Autodesk Fusion 360 part; units mm, degrees
sketch "Sketch3" plane through (0, 0, 18) normal (0, 0, 1) x (1, 0, 0)
  line L0 (-33.9, 6.35) -> (-19.5, 6.35) construction
  line L1 (-19.5, 6.35) -> (-19.5, -6.35) construction
  line L2 (-19.5, -6.35) -> (-33.9, -6.35) construction
  line L3 (-33.9, -6.35) -> (-33.9, 6.35) construction
  line L4 (19.5, 6.35) -> (33.9, 6.35) construction
  line L5 (33.9, 6.35) -> (33.9, -6.35) construction
  line L6 (33.9, -6.35) -> (19.5, -6.35) construction
  line L7 (19.5, -6.35) -> (19.5, 6.35) construction
  line L8 (-35.9, 8.35) -> (35.9, 8.35)
  line L9 (35.9, 8.35) -> (35.9, -8.35)
  line L10 (35.9, -8.35) -> (-35.9, -8.35)
  line L11 (-35.9, -8.35) -> (-35.9, 8.35)
  line L12 (-35.9, 8.35) -> (35.9, -8.35) construction
  line L13 (34, 6.45) -> (34, -6.45)
  line L14 (34, -6.45) -> (19.4, -6.45)
  line L15 (19.4, -6.45) -> (19.4, 6.45)
  line L16 (19.4, 6.45) -> (34, 6.45)
  line L17 (-19.4, -6.45) -> (-34, -6.45)
  line L18 (-34, -6.45) -> (-34, 6.45)
  line L19 (-34, 6.45) -> (-19.4, 6.45)
  line L20 (-19.4, 6.45) -> (-19.4, -6.45)
  dimension "d5" = 14.4
  dimension "d6" = 12.7
  dimension "d7" = 14.4
  dimension "d8" = 12.7
  dimension "d9" = 39
  dimension "d12" = 2
  dimension "d13" = 2
  dimension "d15" = 2
  dimension "d16" = 2
extrude "Extrude3" add sketch "Sketch3" along normal blind 18
sketch "Sketch4" plane through (0, 8.35, 0) normal (0, 1, 0) x (-1, 0, 0)
  line L0 (-35.9, 18) -> (35.9, 18)
  line L1 (35.9, 18) -> (35.9, 36)
  line L2 (35.9, 36) -> (-35.9, 36)
  line L3 (-35.9, 36) -> (-35.9, 18)
  circle A0 centre (27.55, 22) radius 2.075
  circle A1 centre (27.55, 32) radius 2.075
  line L4 (35.9, 27) -> (-35.9, 27) construction
  line L5 (34, 18) -> (34, 36)
  line L6 (34, 36) -> (34, 18)
  line L7 (19.4, 18) -> (19.4, 36)
  line L8 (19.4, 36) -> (19.4, 18)
  line L9 (34, 18) -> (19.4, 18) construction
  line L10 (34, 36) -> (19.4, 36) construction
  line L11 (27.55, 18) -> (27.55, 36)
  line L12 (0, 18) -> (0, 36) construction
  circle A2 centre (-27.55, 22) radius 2.075
  circle A3 centre (-27.55, 32) radius 2.075
  line L13 (26.7, 18) -> (26.7, 36) construction
  point P0 (27.55, 18)
  point P1 (27.55, 36)
  dimension "d19" = 4.15
  dimension "d22" = 10
  dimension "d23" = 5
  dimension "d48" = 6.45
extrude "Extrude4" cut sketch "Sketch4" against normal blind 16.7 contours A0 L11 | A0 L11 | A1 L11 | A1 L11 | A2 | A3
sketch "Sketch5" plane through (0, 8.35, 0) normal (0, 1, 0) x (-1, 0, 0)
  circle A0 centre (27.55, 32) radius 2.075
  circle A1 centre (27.55, 22) radius 2.075
  line L0 (-35.9, 18) -> (35.9, 18)
  line L1 (35.9, 18) -> (35.9, 36)
  line L2 (35.9, 36) -> (-35.9, 36)
  line L3 (-35.9, 36) -> (-35.9, 18)
  line L4 (35.9, 27) -> (-35.9, 27) construction
  line L5 (0, 18) -> (0, 36) construction
  line L6 (-6.35, 20.65) -> (6.35, 20.65) construction
  line L7 (6.35, 20.65) -> (6.35, 33.35) construction
  line L8 (6.35, 33.35) -> (-6.35, 33.35) construction
  line L9 (-6.35, 33.35) -> (-6.35, 20.65) construction
  line L10 (-6.35, 20.65) -> (6.35, 33.35) construction
  line L11 (6.35, 20.65) -> (-6.35, 33.35) construction
  circle A2 centre (-27.55, 22) radius 2.075
  circle A3 centre (-27.55, 32) radius 2.075
  line L12 (-6.45, 33.45) -> (-6.45, 20.55)
  line L13 (-6.45, 20.55) -> (6.45, 20.55)
  line L14 (6.45, 20.55) -> (6.45, 33.45)
  line L15 (6.45, 33.45) -> (-6.45, 33.45)
  point P0 (0, 27)
  dimension "d27" = 12.7
  dimension "d28" = 12.7
  dimension "d40" = 0.1
extrude "Extrude5" cut sketch "Sketch5" against normal blind 16.7 contours L12 L13 L14 L15
sketch "Sketch6" plane through (0, 0, 36) normal (0, 0, 1) x (1, 0, 0)
  line L0 (-35.9, -8.35) -> (35.9, -8.35)
  line L1 (35.9, -8.35) -> (35.9, 8.35)
  line L2 (35.9, 8.35) -> (-35.9, 8.35)
  line L3 (-35.9, 8.35) -> (-35.9, -8.35)
  line L4 (6.45, 0) -> (-6.45, 0) construction
  circle A0 centre (0, 5) radius 2.075
  circle A1 centre (0, -5) radius 2.075
  line L5 (-34, 6.45) -> (-19.4, 6.45)
  line L6 (-19.4, 6.45) -> (-19.4, -6.45)
  line L7 (-19.4, -6.45) -> (-34, -6.45)
  line L8 (-34, -6.45) -> (-34, 6.45)
  line L9 (19.4, -6.45) -> (19.4, 6.45)
  line L10 (19.4, 6.45) -> (34, 6.45)
  line L11 (34, 6.45) -> (34, -6.45)
  line L12 (34, -6.45) -> (19.4, -6.45)
  line L13 (-6.45, 8.35) -> (6.45, 8.35)
  line L14 (6.45, 8.35) -> (6.45, -8.35)
  line L15 (6.45, -8.35) -> (-6.45, -8.35)
  line L16 (-6.45, -8.35) -> (-6.45, 8.35)
  line L17 (0, 8.35) -> (0, -8.35) construction
  dimension "d31" = 4.15
  dimension "d32" = 10
  dimension "d33" = 5
extrude "Extrude6" cut sketch "Sketch6" against normal blind 18 contours A0 | A1
equation "d5 = 12.7 mm + addl_wire_space"
equation "d7 = 12.7 mm + addl_wire_space"
equation "d19 = 4 mm + tolerance_hole"
equation "d31 = 4 mm + tolerance_hole"
equation "tolerance_bar = 0.1 mm"
equation "tolerance_hole = 0.15 mm"
equation "d40 = tolerance_bar"
equation "addl_wire_space = 0.9 mm + 0.8 mm"
equation "d48 = 12.7 mm / 2 + tolerance_bar"
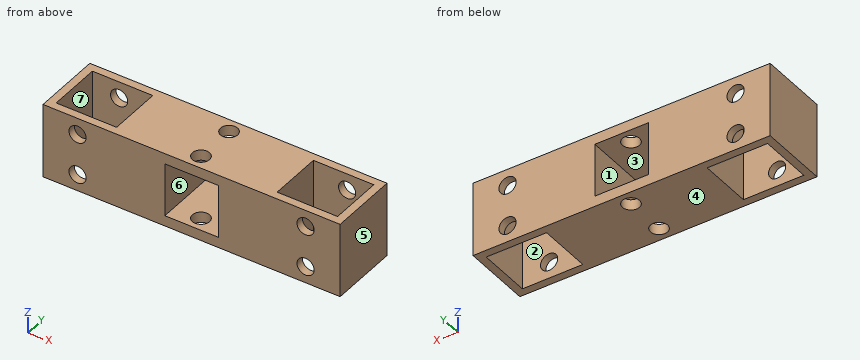
Work out the finished part from the listing and answer in its coordinate system (mm). Face numbers are marked on the shaded views. A direction names the side the tool comes from. Give positions to 0.01 mm unless a question says otherwise; leave off trailing zeros. Write each loop counter-clockwise with the first axis right and the second up, starting at its lowest first coordinate (ties: lowest second). Pieces come first, ordered by that corner, then holes. Notation, with made-up numbers: (58, -36) -> (116, -36) arc R32 ccw to (116, -8) -> close; hole circle Ø8 at (-33, 0.25). An arc over 180 degrees is marked (long way). Write item = value, one per line.
Q1. Section A-A on y = -1.25 is taken. Determine the outline of the cut face in (x, z).
Computed values:
outline = (-35.9, 18) -> (-34, 18) -> (-34, 36) -> (-35.9, 36) -> close; (-19.4, 18) -> (19.4, 18) -> (19.4, 36) -> (-19.4, 36) -> close; (34, 18) -> (35.9, 18) -> (35.9, 36) -> (34, 36) -> close; hole (-6.45, 20.55) -> (6.45, 20.55) -> (6.45, 33.45) -> (-6.45, 33.45) -> close
Q2. Section B-B on z = 27.25 is taken. Determine the outline of the cut face in (x, y), and give its area (3 significant figures).
Computed values:
outline = (-35.9, -8.35) -> (-6.45, -8.35) -> (-6.45, 8.35) -> (-35.9, 8.35) -> close; (6.45, -8.35) -> (35.9, -8.35) -> (35.9, 8.35) -> (6.45, 8.35) -> close; hole (-34, -6.45) -> (-19.4, -6.45) -> (-19.4, 6.45) -> (-34, 6.45) -> close; hole (19.4, -6.45) -> (34, -6.45) -> (34, 6.45) -> (19.4, 6.45) -> close
area = 607 mm^2
Q3. For a pull along Z with two mould halves and no side action, classify the marked faces 1, 2, 3 and 4 as pulls with the +Z half, pulls with the -Z half, needs draft (parallel to the pull), parting line crosses it, or undercut.
Computed values:
face_1 = undercut
face_2 = needs draft
face_3 = undercut
face_4 = pulls with the -Z half
Q4. Section C-C on y = -5 is taken. Determine the outline of the cut face in (x, z) (3 decimals).
Computed values:
outline = (-35.9, 18) -> (-34, 18) -> (-34, 36) -> (-35.9, 36) -> close; (-19.4, 18) -> (-2.075, 18) -> (-2.075, 20.55) -> (-6.45, 20.55) -> (-6.45, 33.45) -> (-2.075, 33.45) -> (-2.075, 36) -> (-19.4, 36) -> close; (2.075, 18) -> (19.4, 18) -> (19.4, 36) -> (2.075, 36) -> (2.075, 33.45) -> (6.45, 33.45) -> (6.45, 20.55) -> (2.075, 20.55) -> close; (34, 18) -> (35.9, 18) -> (35.9, 36) -> (34, 36) -> close
Q5. A flat-ended cylindrical pin translates along its axis: pin 1 Ø2.5 at (x, y) = (0, -5) entering from -Z. Find the tip coordinate at first contact, or state that the pin passes through.
Computed values:
pin_1 = through
Q6. Section D-D on x = -27.55 is taken. Determine the outline of the cut face in (y, z) (3 decimals).
Computed values:
outline = (-8.35, 18) -> (-6.45, 18) -> (-6.45, 19.925) -> (-8.35, 19.925) -> close; (-8.35, 24.075) -> (-6.45, 24.075) -> (-6.45, 29.925) -> (-8.35, 29.925) -> close; (-8.35, 34.075) -> (-6.45, 34.075) -> (-6.45, 36) -> (-8.35, 36) -> close; (6.45, 18) -> (8.35, 18) -> (8.35, 19.925) -> (6.45, 19.925) -> close; (6.45, 24.075) -> (8.35, 24.075) -> (8.35, 29.925) -> (6.45, 29.925) -> close; (6.45, 34.075) -> (8.35, 34.075) -> (8.35, 36) -> (6.45, 36) -> close
Q7. A tool of negligible diameter and unlimited length cuts with its end or side. For the marked faces 5, 6 and 7, from which of +Z, -Z, +X, -X, +Y, -Y can it reach the whole face along a straight path? Write none if from no direction.
Computed values:
face_5 = +Z, -Z, +X, +Y, -Y
face_6 = +Y, -Y
face_7 = +Z, -Z
Q8. Consider line 1 along Z through (x, y) = (27.55, 7.7) (3 decimals); line 2 along X through (y, z) = (0, 20.5); line 3 along X through (y, z) = (1.5, 28.5). Determine where each line is inside the solid, lowest interval first.
Computed values:
line_1 = 18 to 19.925, 24.075 to 29.925, 34.075 to 36
line_2 = -35.9 to -34, -19.4 to 19.4, 34 to 35.9
line_3 = -35.9 to -34, -19.4 to -6.45, 6.45 to 19.4, 34 to 35.9
